Autodesk Inventor part; units mm, degrees
ref_plane "YZ Plane" through (0, 0, 0) normal (1, 0, 0) x (0, 1, 0)
ref_plane "XZ Plane" through (0, 0, 0) normal (0, 1, 0) x (-1, 0, 0)
ref_plane "XY Plane" through (0, 0, 0) normal (0, 0, 1) x (1, 0, 0)
sketch "Sketch1" plane through (0, 0, 0) normal (0, 0, 1) x (1, 0, 0)
  line L0 (0, 0) -> (-1.25, 0)
  line L1 (-1.25, 0) -> (-1.25, 5)
  line L2 (-1.25, 5) -> (-1.15, 5)
  line L3 (-1.15, 5) -> (-1.15, 6)
  line L4 (-1.15, 6) -> (-2.25, 6)
  line L5 (-2.25, 6) -> (-2.25, 7.6)
  line L6 (-2.25, 7.6) -> (0, 7.6)
  line L7 (0, 7.6) -> (0, 0)
  dimension "d0" = 1.6
  dimension "d1" = 2.25
  dimension "d2" = 1.25
  dimension "d3" = 0.1
  dimension "d4" = 1
  dimension "d5" = 7.6
  dimension "d6" = 90
revolve "Revolution1" add sketch "Sketch1" angle 360 about axis through (0, 7.6, 0) along (0, -1, 0)
thread "Thread1"
sketch "Sketch2" plane through (0, 7.6, 0) normal (0, 1, 0) x (1, 0, 0)
  line L0 (5, 0.3) -> (-5, 0.3)
  line L1 (-5, 0.3) -> (-5, -0.3)
  line L2 (-5, -0.3) -> (5, -0.3)
  line L3 (5, -0.3) -> (5, 0.3)
  line L4 (5, 0.3) -> (-5, -0.3) construction
  line L5 (-5, 0.3) -> (5, -0.3) construction
  point P0 (0, 0)
  dimension "d10" = 10
  dimension "d11" = 0.6
fillet "Fillet1" radius 0.25 1 edges at (2.25, 7.6, 0)
extrude "Extrusion2" cut sketch "Sketch2" against normal blind 0.7
fillet "Fillet2" radius 0.3 1 edges at (1.15, 6, 0)
properties part number "Screw-CheeseHead-Brass-M2.5x08" material "Brass, Soft Yellow"
Read the model definition and answer for the solid it produces. Units are mm, in the model's axes. Give positions to 0.01 mm unless a question says otherwise; leave off trailing zeros. Loops run counter-clockwise (first coordinate to the right, second up) from the corner with the lowest first, then second, coordinate; pieces in that order, holes last. Notation, with made-up numbers: (-20, 45) - (26, 45) arc R14 ccw to (26, 63) - close; hole circle Ø2 at (-6, 65.5). An arc over 180 degrees is marked (long way). Answer as CSV lines item,"result". Start each with the question number.
1) Each of these flat-tipped pins is pushed along its axis until it touches: pin 1 Ø2 at (x, y) = (0.5, 3.5) entering from +Z; pin 2 Ø1.2 at (x, z) = (0, 0) entering from +Y; pin 3 Ø0.8 at (x, y) = (-1, 7.5) entering from +Z; pin 4 Ø0.6 at (x, y) = (1, 7.5) entering from -Z. Where does it stop, or does it pass through?
2) Determine the mould class of faces 1 (the face through (0, 7.6, 1)), 2 (the face through (0.27, 2.54, -1.22)), 3 (the face through (0, 0, 0)), 4 (the face through (0.91, 5.35, -0.7)) for opening direction Y: released by +Y, released by -Y, zero draft, split by the parting line, or undercut.
3) Straight lines are drawn through the part: L1, parallel to Z at x = 0.3, y = 6.75; L2, parallel to Y at x = -0.6, z = 0; L3, parallel to Y at x = 1.25, z = -1.2. For each, find the intervals that lie inside material, in ascending order. Write a range as from..to.
4) Find section B-B (z = 0). Write down the section's boundary in (x, y), then the cut area to 3 significant figures.
5) Find section A-A (x = 0). Write down the section's boundary in (y, z).
6) Find section C-C (y = 1.75). Write down the section's boundary in (x, z), then the cut area to 3 significant figures.
Findings below:
1,pin 1,"z = 1.25"
1,pin 2,"y = 7.6"
1,pin 3,"z = 2.16"
1,pin 4,"z = -2.13"
2,face 1,"released by +Y"
2,face 2,"zero draft"
2,face 3,"released by -Y"
2,face 4,"undercut"
3,L1,"-2.23..2.23"
3,L2,"0..6.9"
3,L3,"6..7.6"
4,outline,"(-2.25, 6) - (-1.45, 6) arc R0.3 cw to (-1.15, 5.7) - (-1.15, 5) - (-1.25, 5) - (-1.25, 0) - (1.25, 0) - (1.25, 5) - (1.15, 5) - (1.15, 5.7) arc R0.3 cw to (1.45, 6) - (2.25, 6) - (2.25, 6.9) - (-2.25, 6.9) - close"
4,area,"18.9 mm^2"
5,outline,"(0, -1.25) - (5, -1.25) - (5, -1.15) - (5.7, -1.15) arc R0.3 cw to (6, -1.45) - (6, -2.25) - (7.35, -2.25) arc R0.25 ccw to (7.6, -2) - (7.6, -0.3) - (6.9, -0.3) - (6.9, 0.3) - (7.6, 0.3) - (7.6, 2) arc R0.25 ccw to (7.35, 2.25) - (6, 2.25) - (6, 1.45) arc R0.3 cw to (5.7, 1.15) - (5, 1.15) - (5, 1.25) - (0, 1.25) - close"
6,outline,"circle Ø2.5 at (0, 0)"
6,area,"4.91 mm^2"
